Design review of the part built by this model. Coordinates are the model's own, in mm. Face numbers are marked on the shaded views. Coordinates: 2 decimals unless noted, no trailing zeros. Order: outer loops, then holes, each group sorted by start corner. A loop starts at its lowest first (then second) coordinate and runs counter-clockwise, first axis right, second up. Notation, with made-up numbers: M 20.25,38 L 58.25,38 A14 cw 58.25,61 Z; hole C -39.5,24 d5. An arc over 180 degrees is marked long. Answer as a JSON object with one key per item and string values.
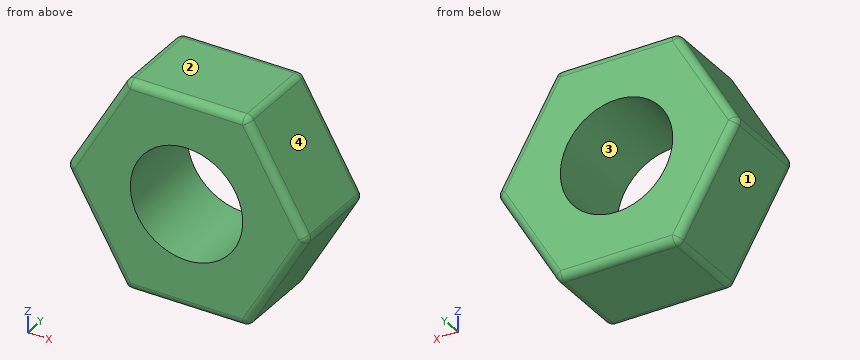
Autodesk Inventor part; units mm, degrees
ref_plane "YZ Plane" through (0, 0, 0) normal (1, 0, 0) x (0, 1, 0)
ref_plane "XZ Plane" through (0, 0, 0) normal (0, 1, 0) x (-1, 0, 0)
ref_plane "XY Plane" through (0, 0, 0) normal (0, 0, 1) x (1, 0, 0)
sketch "Sketch1" plane through (0, 0, 0) normal (0, 1, 0) x (-1, 0, 0)
  line L0 (3.1466, 0) -> (1.5733, -2.725)
  line L1 (1.5733, -2.725) -> (-1.5733, -2.725)
  line L2 (-1.5733, -2.725) -> (-3.1466, 0)
  line L3 (-3.1466, 0) -> (-1.5733, 2.725)
  line L4 (-1.5733, 2.725) -> (1.5733, 2.725)
  line L5 (1.5733, 2.725) -> (3.1466, 0)
  circle A0 centre (0, 0) radius 1.465
  dimension "d0" = 5.45
  dimension "d1" = 2.93
extrude "Extrusion1" add sketch "Sketch1" along normal blind 2.42
fillet "Fillet1" radius 0.2 18 edges at (2.3599, 2.42, 1.3625) (0, 2.42, 2.725) (1.5733, 1.21, 2.725) (0, 0, 2.725) (-1.5733, 1.21, 2.725) (2.3599, 0, 1.3625) (3.1466, 1.21, 0) (1.5733, 1.21, -2.725) (2.3599, 2.42, -1.3625) (2.3599, 0, -1.3625) (-1.5733, 1.21, -2.725) (0, 2.42, -2.725) (0, 0, -2.725) (-2.3599, 2.42, 1.3625) (-2.3599, 2.42, -1.3625) (-3.1466, 1.21, 0) (-2.3599, 0, -1.3625) (-2.3599, 0, 1.3625)
thread "Thread1"
properties part number "M3 Nut"
1) Add section B-B (x = 0). State the section outline as (y, z) points (3 decimals).
Taken from the geometry:
{"outline": "M 0,-2.525 A0.2 ccw 0.2,-2.725 L 2.22,-2.725 A0.2 ccw 2.42,-2.525 L 2.42,-1.465 L 0,-1.465 Z; M 0,1.465 L 2.42,1.465 L 2.42,2.525 A0.2 ccw 2.22,2.725 L 0.2,2.725 A0.2 ccw 0,2.525 Z"}
2) To check wall thickness, follow L1, parallel to Z at x = 0, y = 1.85 (3 decimals); L2, parallel to Z at x = -1, y = 0.95 (3 decimals); L3, parallel to X at y = 1.75, z = 0.3. State the ranges of each line that lie inside material, in increasing order.
Taken from the geometry:
{"L1": "z = -2.725 to -1.465, 1.465 to 2.725", "L2": "z = -2.725 to -1.071, 1.071 to 2.725", "L3": "x = -2.97 to -1.43, 1.43 to 2.97"}
3) Mouldability with a two-part tool opening along X and no side actions: class the marked faces 1, 2, 3 and 4 as released by +X, released by -X, zero draft, split by the parting line, or undercut.
Taken from the geometry:
{"face 1": "released by -X", "face 2": "zero draft", "face 3": "undercut", "face 4": "released by +X"}
4) Add section C-C (x = -1). State the section outline as (y, z) points (3 decimals).
Taken from the geometry:
{"outline": "M 0,-2.525 A0.2 ccw 0.2,-2.725 L 2.22,-2.725 A0.2 ccw 2.42,-2.525 L 2.42,-1.071 L 0,-1.071 Z; M 0,1.071 L 2.42,1.071 L 2.42,2.525 A0.2 ccw 2.22,2.725 L 0.2,2.725 A0.2 ccw 0,2.525 Z"}
5) Add section A-A (y = 0.4). State the section outline as (x, z) points (3 decimals), and give its area (3 significant figures).
Taken from the geometry:
{"outline": "M -3.089,-0.1 L -1.631,-2.625 A0.2 ccw -1.458,-2.725 L 1.458,-2.725 A0.2 ccw 1.631,-2.625 L 3.089,-0.1 A0.2 ccw 3.089,0.1 L 1.631,2.625 A0.2 ccw 1.458,2.725 L -1.458,2.725 A0.2 ccw -1.631,2.625 L -3.089,0.1 A0.2 ccw Z; hole C 0,0 d2.93", "area": "19.0 mm2"}
